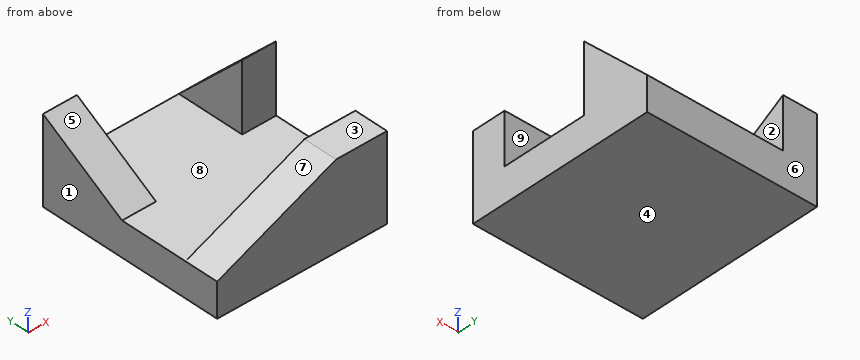
Autodesk Inventor part; units mm, degrees
ref_plane "YZ Plane" through (0, 0, 0) normal (1, 0, 0) x (0, 1, 0)
ref_plane "XZ Plane" through (0, 0, 0) normal (0, 1, 0) x (-1, 0, 0)
ref_plane "XY Plane" through (0, 0, 0) normal (0, 0, 1) x (1, 0, 0)
sketch "Sketch1" plane through (0, 0, 0) normal (0, 0, 1) x (1, 0, 0)
  line L0 (-23.0214, 29.9269) -> (26.9786, 29.9269)
  line L1 (26.9786, 29.9269) -> (26.9786, -25.0731)
  line L2 (26.9786, -25.0731) -> (-23.0214, -25.0731)
  line L3 (-23.0214, -25.0731) -> (-23.0214, 29.9269)
  point P0 (0, 0)
  dimension "d0" = 55
  dimension "d1" = 50
  dimension "d4" = 55
  dimension "d5" = 50
extrude "Extrusion1" add sketch "Sketch1" along normal blind 10
ref_plane "Work Plane1" through (-23.0214, -25.0731, 0) normal (-1, 0, 0) x (0, 0, 1)
sketch "Sketch3" plane through (-23.0214, -25.0731, 0) normal (-1, 0, 0) x (0, 0, 1)
  line L0 (10, 0) -> (10, 55)
  line L1 (10, 55) -> (25, 55)
  line L2 (25, 55) -> (9.9866, 30.0136)
  line L3 (10, 55) -> (9.9866, 30.0136)
  line L4 (10, 55) -> (9.9866, 30.0136)
  point P0 (0, 25.0731)
  point P1 (10, 30.0358)
  dimension "d10" = 15
  dimension "d14" = 29.15
  dimension "d15" = 59
  dimension "d16" = 55
extrude "Extrusion2" add sketch "Sketch3" against normal blind 10 contours L0 L1 L2
ref_plane "Work Plane2" through (26.9786, -25.0731, 0) normal (1, 0, 0) x (0, 0, -1)
sketch "Sketch4" plane through (26.9786, -25.0731, 0) normal (1, 0, 0) x (0, 0, -1)
  line L0 (-10, 0) -> (-10, 55)
  line L1 (-10, 35) -> (-30, 35)
  line L2 (-30, 35) -> (-10, 55)
  line L3 (-10, 55) -> (-10, 35)
  point P0 (0, 25.0731)
  dimension "d20" = 20
  dimension "d21" = 20
  dimension "d22" = 28.2843
  dimension "d23" = 45
extrude "Extrusion3" add sketch "Sketch4" against normal blind 10
ref_plane "Work Plane3" through (-23.0214, -25.0731, 0) normal (0, -1, 0) x (1, 0, 0)
sketch "Sketch5" plane through (-23.0214, -25.0731, 0) normal (0, -1, 0) x (1, 0, 0)
  line L0 (50, 0) -> (50, 10)
  line L1 (50, 10) -> (50, 25)
  line L2 (50, 25) -> (35, 25)
  line L3 (35, 25) -> (0, 10)
  line L4 (0, 10) -> (50, 10)
  point P0 (23.0214, 0)
  point P1 (0, 25)
  dimension "d27" = 15
  dimension "d28" = 15
  dimension "d29" = 38.0789
  dimension "d30" = 35
extrude "Extrusion4" add sketch "Sketch5" against normal blind 10
Geometry check sheet. Reference: the model listing, model coordinates, mm. Face numbers are marked on the shaded views. A direction names the side the tool comes from. Give positions to 0.01 mm unless a question says otherwise; leave off trailing zeros. Loops run counter-clockwise (first coordinate to the right, second up) from the corner with the lowest first, then second, coordinate; pieces in that order, holes last.
(1) Section check A-A on x = 14. Record the cut outline in (y, z).
From the geometry:
outline: (-25.07, 0) - (29.93, 0) - (29.93, 10) - (-15.07, 10) - (-15.07, 25) - (-25.07, 25) - close
(2) Thickness scan on L1, parallel to X at y = 23, z = 16.5; L2, parallel to Y at x = 4.5, z = 14.25; L3, parallel to Z at x = -16, y = -11.5. Record the ranges inside material, lowest first.
From the geometry:
L1: x = -23.02 to -13.02, 16.98 to 26.98
L2: y = -25.07 to -15.07
L3: z = 0 to 10
(3) Section check C-C on y = 13. Record the cut outline in (x, z).
From the geometry:
outline: (-23.02, 0) - (26.98, 0) - (26.98, 26.93) - (16.98, 26.93) - (16.98, 10) - (-13.02, 10) - (-13.02, 14.83) - (-23.02, 14.83) - close
(4) Set-up check for the marked faces 1, 2, 3, 4 and 5: record each of +Z, -Z, +X, -X, +Y, -Y from which the full face is reachable in a straight line by a thin tool's end or side.
From the geometry:
face 1: +Z, -Z, -X, +Y, -Y
face 2: +Z, +Y
face 3: +Z, +X, -X, -Y
face 4: -Z, +X, -X, +Y, -Y
face 5: +Z, -X
(5) Release check for a two-part mould opening along Y. For the marked faces 6, 7, 8 and 9 record: released by +Y, released by -Y, zero draft, split by the parting line, or undercut.
From the geometry:
face 6: released by +Y
face 7: zero draft
face 8: undercut
face 9: undercut
(6) Depth check by flat-ended pin: pin 1 Ø5 at (x, y) = (19.5, -22) entering from +Z; pin 2 Ø4.5 at (x, z) = (1.5, 20.5) entering from +Y; pin 3 Ø8 at (x, y) = (17.5, 17.5) entering from +Z. Enter the tip coordinate at first touch or a pass-through.
From the geometry:
pin 1: stops at z = 25
pin 2: stops at y = -15.07
pin 3: stops at z = 26.43
(7) Section check B-B on z = 11. Record the cut outline in (x, y).
From the geometry:
outline: (-23.02, 6.63) - (-13.02, 6.63) - (-13.02, 29.93) - (-23.02, 29.93) - close; (-20.69, -25.07) - (26.98, -25.07) - (26.98, -15.07) - (-20.69, -15.07) - close; (16.98, 9.93) - (26.98, 9.93) - (26.98, 28.93) - (16.98, 28.93) - close
(8) Section check D-D on z = 22.5. Record the cut outline in (x, y).
From the geometry:
outline: (-23.02, 25.77) - (-13.02, 25.77) - (-13.02, 29.93) - (-23.02, 29.93) - close; (6.15, -25.07) - (26.98, -25.07) - (26.98, -15.07) - (6.15, -15.07) - close; (16.98, 9.93) - (26.98, 9.93) - (26.98, 17.43) - (16.98, 17.43) - close
